Check sheet for the modelled part. Datum: model origin and axes. Units: mm. A direction names the side the tool comes from. Coordinates: 2 decimals unless noted, no trailing zeros. Loops run counter-clockwise (first coordinate to the right, second up) from the corner with the lowest first, then second, coordinate; pieces in that order, holes last. Notation, with made-up numbers: (70, 52.25) -> (112, 52.25) arc R15 cw to (112, 63.25) -> close; hole circle Ø9 at (-35.5, 18.5). An arc over 180 degrees is marked (long way). Use one line per item in the form item = value.
from build123d import *

# Parameters (mm, degrees)
BOSS_EXTRUDE1_DEPTH                         = 60
FILLET1_R                                   = 1
TAPPED_START                                = -7
TAPPED_HOLE_FOR_M2_5X0_45_HELICOIL1_OUTL_R  = 1.275
TAPPED_HOLE_FOR_M2_5X0_45_HELICOIL1_DEPTH   = 7
TAPPED_START_2                              = -8.425
TAPPED_HOLE_FOR_M2_5X0_45_HELICOIL1_2_OU_R  = 1.275
TAPPED_HOLE_FOR_M2_5X0_45_HELICOIL1_2_DEPTH = 1.425


# Read off the part's stored shape, not the designer's step: Tapped Hole for M2.5x0.45 Helicoil1
with BuildPart() as part:
    # Sketch1 → Boss-Extrude1 (new body)
    with BuildSketch(Plane.XY):
        with BuildLine():
            Line((0, 0), (8.225, 0))
            Line((8.225, 0), (8.225, -1.25))
            ThreePointArc((8.225, -1.25), (15.833583974, -10.821735736), (26.875, -5.568564576))
            Line((26.875, -5.568564576), (28.875, -5.568564576))
            ThreePointArc((28.875, -5.568564576), (39.831080274, -10.841095968), (47.523441352, -1.425))
            Line((47.523441352, -1.425), (51.476558648, -1.425))
            ThreePointArc((51.476558648, -1.425), (59.168919726, -10.841095968), (70.125, -5.568564576))
            Line((70.125, -5.568564576), (72.125, -5.568564576))
            ThreePointArc((72.125, -5.568564576), (83.166416026, -10.821735736), (90.775, -1.25))
            Line((90.775, -1.25), (90.775, 0))
            Line((90.775, 0), (99, 0))
            Line((99, 0), (99, -1.6))
            Line((99, -1.6), (95.52, -1.6))
            Line((95.52, -1.6), (95.52, -7))
            Line((95.52, -7), (91.282866253, -7))
            ThreePointArc((91.282866253, -7), (82.611549593, -12.957684568), (72.625, -9.647916408))
            Line((72.625, -9.647916408), (69.625, -9.647916408))
            ThreePointArc((69.625, -9.647916408), (60.486058022, -13.046953991), (51.90053193, -8.425))
            Line((51.90053193, -8.425), (47.09946807, -8.425))
            ThreePointArc((47.09946807, -8.425), (38.513941978, -13.046953991), (29.375, -9.647916408))
            Line((29.375, -9.647916408), (26.375, -9.647916408))
            ThreePointArc((26.375, -9.647916408), (16.388450407, -12.957684568), (7.717133747, -7))
            Line((7.717133747, -7), (3.48, -7))
            Line((3.48, -7), (3.48, -1.6))
            Line((3.48, -1.6), (0, -1.6))
            Line((0, -1.6), (0, 0))
        make_face()
    extrude(amount=BOSS_EXTRUDE1_DEPTH)

    # Fillet1
    fillet1_edges = [part.edges().sort_by_distance(p)[0] for p in [
        (95.52, -1.6, 30),
        (91.282866253, -7, 30),
        (7.717133747, -7, 30),
        (3.48, -1.6, 30),
    ]]
    fillet(fillet1_edges, radius=FILLET1_R)

    # Tapped Hole for M2.5x0.45 Helicoil1 outl → Tapped Hole for M2.5x0.45 Helicoil1 (cut)
    with BuildSketch(Plane(origin=(0, 0, 0), x_dir=(1, 0, 0), z_dir=(0, 1, 0)).offset(TAPPED_START)):
        with Locations((93.02, -15)):
            Circle(TAPPED_HOLE_FOR_M2_5X0_45_HELICOIL1_OUTL_R)
        with Locations((93.02, -45)):
            Circle(TAPPED_HOLE_FOR_M2_5X0_45_HELICOIL1_OUTL_R)
        with Locations((49.5, -15)):
            Circle(TAPPED_HOLE_FOR_M2_5X0_45_HELICOIL1_OUTL_R)
        with Locations((49.5, -45)):
            Circle(TAPPED_HOLE_FOR_M2_5X0_45_HELICOIL1_OUTL_R)
    tapped_hole_for_m2_5x0_45_helicoil1 = extrude(amount=TAPPED_HOLE_FOR_M2_5X0_45_HELICOIL1_DEPTH, mode=Mode.SUBTRACT)

    # Tapped Hole for M2.5x0.45 Helicoil1 2 ou → Tapped Hole for M2.5x0.45 Helicoil1 2 (cut)
    with BuildSketch(Plane(origin=(0, 0, 0), x_dir=(1, 0, 0), z_dir=(0, 1, 0)).offset(TAPPED_START_2)):
        with Locations((49.5, -15)):
            Circle(TAPPED_HOLE_FOR_M2_5X0_45_HELICOIL1_2_OU_R)
        with Locations((49.5, -45)):
            Circle(TAPPED_HOLE_FOR_M2_5X0_45_HELICOIL1_2_OU_R)
    tapped_hole_for_m2_5x0_45_helicoil1_2 = extrude(amount=TAPPED_HOLE_FOR_M2_5X0_45_HELICOIL1_2_DEPTH, mode=Mode.SUBTRACT)

    # Mirror1: Tapped Hole for M2.5x0.45 Helicoil1, Tapped Hole for M2.5x0.45 Helicoil1 2 across plane
    add(tapped_hole_for_m2_5x0_45_helicoil1.mirror(Plane.ZY.offset(-49.5)), mode=Mode.SUBTRACT)
    add(tapped_hole_for_m2_5x0_45_helicoil1_2.mirror(Plane.ZY.offset(-49.5)), mode=Mode.SUBTRACT)


solid = part.part
(1) Scan lines: line 1 along Z through (x, y) = (49.5, -4.5) (3 decimals); line 2 along X through (y, z) = (-1.75, 12); line 3 along X through (y, z) = (-5, 45) (3 decimals). Record each from-to range of solid material in increasing order.
Established:
line_1 = 0 to 13.725, 16.275 to 43.725, 46.275 to 60
line_2 = 3.01 to 8.24, 47.51 to 51.49, 90.76 to 95.99
line_3 = 3.48 to 4.705, 7.255 to 8.969, 46.781 to 48.225, 50.775 to 52.219, 90.031 to 91.745, 94.295 to 95.52
(2) Section check D-D, the plane x = 14.5. Record the boundary of the cut face in (y, z), plus the area to 3 significant figures.
Established:
outline = (-12.53, 0) -> (-10.41, 0) -> (-10.41, 60) -> (-12.53, 60) -> close
area = 127 mm²
(3) Tool access check on faces 4 (the flat face through (71, -5.569, 30)), 5 (the flat face through (28, -9.648, 30)), 6 (the flat face through (98, -1.6, 30)), 7 (the flat face through (95, 0, 30)), 8 (the flat face through (1, -1.6, 30)). Record the directions out of +Z, -Z, +X, -X, +Y, -Y that give a thin tool (end or side, any length) a straight path to the whole face; none if there is none.
Established:
face_4 = +Z, -Z, +Y
face_5 = +Z, -Z, -Y
face_6 = +Z, -Z, +X, -Y
face_7 = +Z, -Z, +X, -X, +Y
face_8 = +Z, -Z, -X, -Y
(4) Section check A-A, the plane x = 93.02. Record the boundary of the cut face in (y, z) (3 decimals).
Established:
outline = (-7, 0) -> (0, 0) -> (0, 13.725) -> (-7, 13.725) -> close; (-7, 16.275) -> (0, 16.275) -> (0, 43.725) -> (-7, 43.725) -> close; (-7, 46.275) -> (0, 46.275) -> (0, 60) -> (-7, 60) -> close
(5) Section check C-C, the plane x = 75.5. Record the boundary of the cut face in (y, z).
Established:
outline = (-11.74, 0) -> (-9.42, 0) -> (-9.42, 60) -> (-11.74, 60) -> close
(6) Mould release check, pull along X, two halves, no side actions. Record for faces 1 (the cylindrical face through (38.654, -13.036, 29.58)), 2 (the flat face through (3.48, -5, 30)), 3 (the flat face through (50, -7, 0)): +X half, -X half, draft (parallel to the pull), parting line (faces both ways), or undercut.
Established:
face_1 = undercut
face_2 = -X half
face_3 = draft
(7) Go/stop test with flat-tipped pins: P1, Ø3.5, axis at x = 71, z = 22.5, coming from the -Y side; P2, Ø4.5, axis at x = 48.5, z = 23.5, coming from the +Y side (3 decimals); P3, Ø1.5, axis at y = -3, z = 9, coming from the -X side; P4, Ø5, axis at x = 67, y = -10.5, coming from the -Z side. Record where each tip stops, or that it passes through.
Established:
P1 = -10
P2 = -1.425
P3 = 3.42
P4 = 0
